Autodesk Fusion 360 part; units mm, degrees
sketch "Sketch1" plane through (0, 0, 0) normal (0, 0, 1) x (1, 0, 0)
  line L0 (0, 48) -> (0, 0)
  line L1 (0, 0) -> (15, 0)
  line L2 (15, 0) -> (15, 30)
  line L3 (30, 45) -> (65, 45)
  line L4 (65, 45) -> (65, 48)
  line L5 (65, 48) -> (0, 48)
  arc A0 (30, 45) -> (15, 30) centre (30, 30) ccw
  arc A1 (30, 45) -> (15, 30) centre (30, 30) ccw
  dimension "d1" = 15
  dimension "d2" = 15
  dimension "d3" = 65
  dimension "d4" = 3
  dimension "d6" = 30
revolve "Revolve1" add sketch "Sketch1" angle 360 about axis through (0, 48, 0) along (0, -1, 0)
hole "Hole1" at (0, 0, 0) direction (0, 1, 0) diameter 26 depth 30 tip angle 150
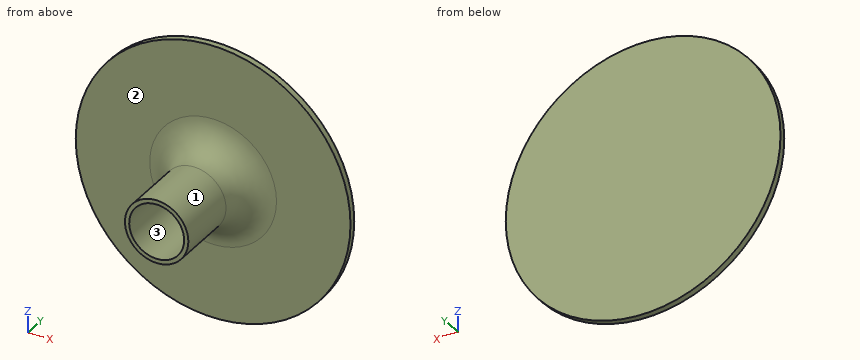
Could you check a few things on this model? Use its own coordinates, in mm. Face numbers are marked on the shaded views. Give positions to 0.01 mm unless a question says otherwise; leave off trailing zeros. Loops run counter-clockwise (first coordinate to the right, second up) from the corner with the lowest first, then second, coordinate; pieces in that order, holes last. Notation, with made-up numbers: (47.5, 44.25) -> (78.5, 44.25) arc R17 cw to (78.5, 71.25) -> close; hole circle Ø7 at (-39, -27.75). An arc over 180 degrees is marked (long way). Return JSON: item names as keys, results as strings.
Item 1: We'd pull the mould along X, two halves only. Please class the marked faces 1, 2 and 3: +X half, -X half, draft (parallel to the pull), parting line (faces both ways), or undercut.
Geometry results:
{"face 1": "parting line", "face 2": "draft", "face 3": "undercut"}
Item 2: I'm going to push flat-ended pins straight in: pin 1 (8 mm diameter, centred on x = 46, z = -40, fed in from -Y); pin 2 (1 mm diameter, centred on x = 0.5, y = 42, fed in from +Z); pin 3 (23.5 mm diameter, centred on x = 0, z = 0, fed in from -Y). Where does each tip first touch, or does it pass through?
Geometry results:
{"pin 1": "stops at y = 45", "pin 2": "stops at z = 21.7", "pin 3": "stops at y = 30.33"}
Item 3: If we section it at C-C on z = 40.5: List the corners of the cut face in (x, y) for me, plus the area to 3 significant figures.
Geometry results:
{"outline": "(-50.84, 45) -> (50.84, 45) -> (50.84, 48) -> (-50.84, 48) -> close", "area": "305 mm²"}
Item 4: If we section it at D-D on y = 39.5: List the corners of the cut face in (x, z) for me, plus the area to 3 significant figures.
Geometry results:
{"outline": "circle Ø36.78 at (0, 0)", "area": "1,060 mm²"}
Item 5: I need wall thicknesses on L1, parallel to Z at x = 0, y = 7.25; L2, parallel to Y at x = -24.5, z = -46; L3, parallel to X at y = 27, z = -12. Which ranges of each line are inside material? Lowest first, please. Write a range as from..to.
Geometry results:
{"L1": "z = -15..-13, 13..15", "L2": "y = 45..48", "L3": "x = -9..-5, 5..9"}
Item 6: If we section it at A-A on y = 17.5: List the corners of the cut face in (x, z) for me, plus the area to 3 significant figures.
Geometry results:
{"outline": "circle Ø30 at (0, 0); hole circle Ø26 at (0, 0)", "area": "176 mm²"}
Item 7: If we section it at B-B on x = -48.5: List the corners of the cut face in (y, z) for me.
Geometry results:
{"outline": "(45, -43.28) -> (48, -43.28) -> (48, 43.28) -> (45, 43.28) -> close"}
